Geometry: see drawing. Coordinates: mm, zero at the bounding-box minimum. Coordinates: 2 decimals unless noted, no trailing zeros. Loops run counter-clockwise (first coordinate to the right, second up) from the corner with the lowest first, then second, coordinate; pieces in that order, holes last. Notation, with made-up numbers: (72, -15) - (84, -15) arc R12 cw to (84, -7) - close; hole circle Ø6 at (-15.75, 33.25). An arc over 180 degrees is marked (long way). Use a Markdown table: item, result. Add a question column.
1. Ray query, L1, parallel to Y at x = 32.5, z = 6.75; L2, parallel to Y at x = 32.5, z = 0.4; L3, parallel to Y at x = 34.5, z = 6.5. Return the intervals inside material, ascending. Write a range as [from, to].
2. Contact query for flat-ended pins moving along their axis: P1, Ø3, axis at x = 50.5, z = 2, coming from the -Y side; P2, Ø4.5, axis at x = 60.28, y = 32.5, coming from the +Z side; P3, Ø2, axis at x = 24, z = 4, coming from the +Y side; P4, Ø2, axis at y = 19.5, z = 2.5, coming from the -X side. Output: stop coordinate, or through.
3. Draft query along X for the marked faces 1, 2 and 3. Return one class per face: released by +X, released by -X, zero draft, split by the parting line, or undercut.
4. Section query C-C on y = 25. Return the cut outline in (x, z) (3 decimals), then the cut area to 3 significant figures.
5. Section query D-D on z = 6.75. Return the cut outline in (x, y).
6. Section query A-A on y = 32.5. Return the cut outline in (x, z), then the cut area to 3 significant figures.
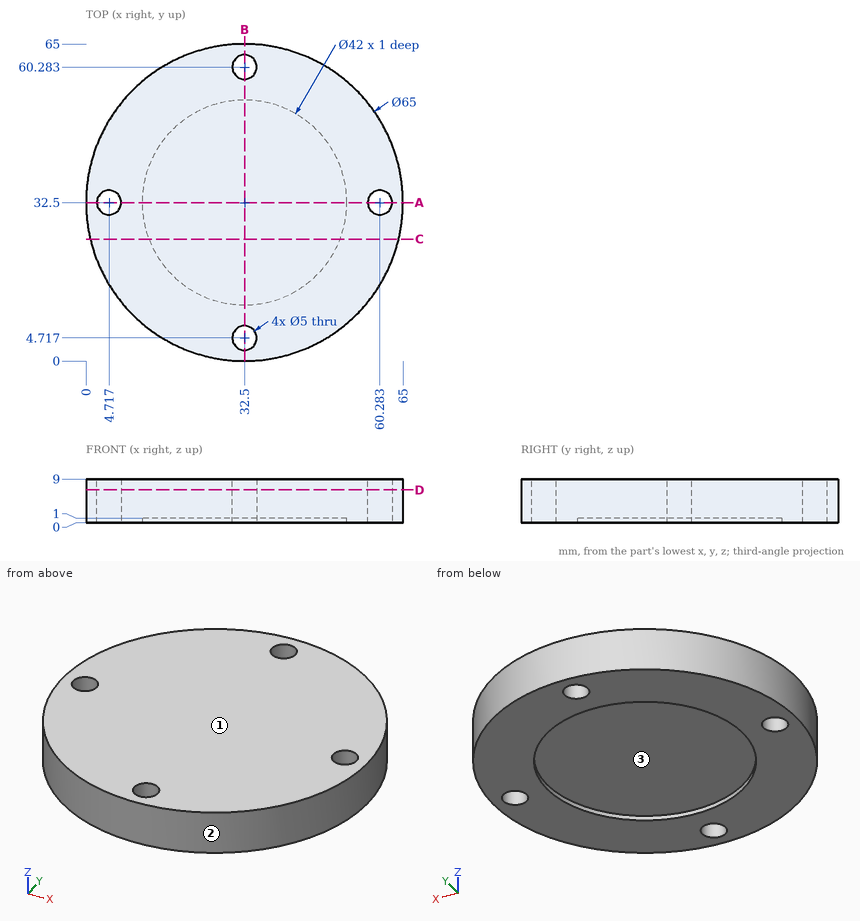
Resolved:
| question | item | result |
|---|---|---|
| 1 | L1 | [0, 2.22], [7.22, 57.78], [62.78, 65] |
| 1 | L2 | [0, 2.22], [7.22, 11.5], [53.5, 57.78], [62.78, 65] |
| 1 | L3 | [0.06, 3.22], [6.22, 58.78], [61.78, 64.94] |
| 2 | P1 | y = 4.5 |
| 2 | P2 | through |
| 2 | P3 | y = 64.12 |
| 2 | P4 | x = 2.3 |
| 3 | face 1 | zero draft |
| 3 | face 2 | split by the parting line |
| 3 | face 3 | undercut |
| 4 | outline | (0.877, 0) - (12.885, 0) - (12.885, 1) - (52.115, 1) - (52.115, 0) - (64.123, 0) - (64.123, 9) - (0.877, 9) - close |
| 4 | area | 530 mm² |
| 5 | outline | circle Ø65 at (32.5, 32.5); hole circle Ø5 at (4.72, 32.5); hole circle Ø5 at (32.5, 4.72); hole circle Ø5 at (32.5, 60.28); hole circle Ø5 at (60.28, 32.5) |
| 6 | outline | (0, 0) - (2.22, 0) - (2.22, 9) - (0, 9) - close; (7.22, 0) - (11.5, 0) - (11.5, 1) - (53.5, 1) - (53.5, 0) - (57.78, 0) - (57.78, 9) - (7.22, 9) - close; (62.78, 0) - (65, 0) - (65, 9) - (62.78, 9) - close |
| 6 | area | 453 mm² |
